The model under review builds one solid part; all positions refer to its coordinate system, in mm. Face numbers are marked on the shaded views. A direction names the side the tool comes from. Give positions to 0.01 mm unless a question says otherwise; leave off trailing zeros. Loops run counter-clockwise (first coordinate to the right, second up) from the corner with the lowest first, then second, coordinate; pieces in that order, holes last. Notation, with made-up numbers: M 26,57 L 53,57 A11 ccw 53,68 Z; hole C 56,-31 d4. An arc over 180 degrees is marked long. Write item = value, one per line. Start each with the question number.
1. We need section A-A on x = 3. Give the boundary of the cut face in (y, z).
2. Wall thickness on line 1 along Y through (x, z) = (2.5, -3.5); line 2 along Z through (x, y) = (6.5, 6.35); line 3 along Y through (x, z) = (10.25, 15.5): over which ranges is each line inside the solid? List them lowest first. Write a range as from..to.
3. Draft analysis for pull direction X (two halves, no side actions). For the marked faces 1, 2 and 3, state which applies: pulls with the +X half, pulls with the -X half, needs draft (parallel to the pull), parting line crosses it, or undercut.
4. For the marked faces 4, 5, 6 and 7, list the 3-axis set-ups (+Z, -Z, +X, -X, +Y, -Y) from which the entire face can be reached by the end or side of a thin tool; tool diameter is ignored.
5. We need section D-D on x = 7. Give the boundary of the cut face in (y, z).
6. We need section C-C on y = 18.5. Give the boundary of the cut face in (x, z).
7. For pin 1 (6.5 mm diameter, centred on x = 6.5, z = -18.14, fed in from -Y); pin 2 (2.5 mm diameter, centred on x = 8, y = 11.5, fed in from +Z); pin 3 (3 mm diameter, centred on x = 3.5, y = -0.5, fed in from -Z), all flat-tipped, find the tip position at first contact; note any pin that passes through.
8. We need section B-B on y = -2. Give the boundary of the cut face in (x, z).
from build123d import *

# Parameters (mm, degrees)
SKETCH2_W           = 29
SKETCH2_H           = 30
SKETCH2_W_2         = 5.4
SKETCH2_H_2         = 3.5
SKETCH2_W_3         = 5.8
SKETCH2_H_3         = 5.3
BOSS_EXTRUDE1_DEPTH = 13
CUT_EXTRUDE1_DEPTH  = 5.3
CUT_EXTRUDE2_DEPTH  = 31
FILLET1_R           = 1


with BuildPart() as part:
    # Sketch2 → Boss-Extrude1 (new body)
    with BuildSketch(Plane(origin=(0, 0, 0), x_dir=(0, 0, -1), z_dir=(1, 0, 0))):
        Rectangle(SKETCH2_W, SKETCH2_H)
        with Locations((-17.2, 5.55)):
            Rectangle(SKETCH2_W_2, SKETCH2_H_2)
        with Locations((4.1, 17.65)):
            Rectangle(SKETCH2_W_3, SKETCH2_H_3)
        with Locations((17.2, 5.55)):
            Rectangle(SKETCH2_W_2, SKETCH2_H_2)
    extrude(amount=BOSS_EXTRUDE1_DEPTH)

    # Sketch3 → Cut-Extrude1 (cut)
    with BuildSketch(Plane(origin=(0, 15, 0), x_dir=(1, 0, 0), z_dir=(0, 1, 0))):
        with BuildLine():
            Line((6.5, 1.2), (9.4, 1.2))
            Line((9.4, 1.2), (9.4, 4.1))
            ThreePointArc((9.4, 4.1), (8.550609665, 2.049390335), (6.5, 1.2))
        make_face()
        with BuildLine():
            ThreePointArc((6.5, 7), (8.550609665, 6.150609665), (9.4, 4.1))
            Line((9.4, 4.1), (9.4, 7))
            Line((9.4, 7), (6.5, 7))
        make_face()
        with BuildLine():
            ThreePointArc((3.6, 4.1), (4.449390335, 6.150609665), (6.5, 7))
            Line((6.5, 7), (3.6, 7))
            Line((3.6, 7), (3.6, 4.1))
        make_face()
        with BuildLine():
            Line((3.6, 1.2), (6.5, 1.2))
            ThreePointArc((6.5, 1.2), (4.449390335, 2.049390335), (3.6, 4.1))
            Line((3.6, 4.1), (3.6, 1.2))
        make_face()
        Polygon((0, 1.2), (3.6, 1.2), (3.6, 4.1), (3.6, 7), (0, 7), align=None)
        Polygon((9.4, 1.2), (13, 1.2), (13, 7), (9.4, 7), (9.4, 4.1), align=None)
        with BuildLine():
            Line((7.75, 19.7), (7.75, 19.9))
            Line((7.75, 19.9), (5.25, 19.9))
            Line((5.25, 19.9), (5.25, 19.7))
            ThreePointArc((5.25, 19.7), (6.5, 16.1387505), (7.75, 19.7))
        make_face()
        with BuildLine():
            Line((5.25, -19.9), (7.75, -19.9))
            Line((7.75, -19.9), (7.75, -19.7))
            ThreePointArc((7.75, -19.7), (6.5, -16.1387505), (5.25, -19.7))
            Line((5.25, -19.7), (5.25, -19.9))
        make_face()
    extrude(amount=CUT_EXTRUDE1_DEPTH, mode=Mode.SUBTRACT)

    # Sketch3<4> → Cut-Extrude2 (cut, through all)
    with BuildSketch(Plane(origin=(0, 15, 0), x_dir=(1, 0, 0), z_dir=(0, 1, 0))):
        with BuildLine():
            Line((7.75, 19.7), (7.75, 19.9))
            Line((7.75, 19.9), (5.25, 19.9))
            Line((5.25, 19.9), (5.25, 19.7))
            ThreePointArc((5.25, 19.7), (6.5, 16.1387505), (7.75, 19.7))
        make_face()
        with BuildLine():
            Line((5.25, -19.9), (7.75, -19.9))
            Line((7.75, -19.9), (7.75, -19.7))
            ThreePointArc((7.75, -19.7), (6.5, -16.1387505), (5.25, -19.7))
            Line((5.25, -19.7), (5.25, -19.9))
        make_face()
    extrude(amount=-CUT_EXTRUDE2_DEPTH, mode=Mode.SUBTRACT)

    # Fillet1
    fillet1_edges = [part.edges().sort_by_distance(p)[0] for p in [
        (0, 5.55, -19.9),
        (0, -5.6, -14.5),
        (0, -15, 0),
        (0, -5.6, 14.5),
        (0, 5.55, 19.9),
        (0, 11.15, 14.5),
        (0, 11.15, -14.5),
        (6.5, -15, -14.5),
        (6.5, -15, 14.5),
        (13, 11.15, 14.5),
        (13, 5.55, 19.9),
        (13, 11.15, -14.5),
        (13, -5.6, 14.5),
        (13, -15, 0),
        (13, -5.6, -14.5),
        (13, 5.55, -19.9),
    ]]
    fillet(fillet1_edges, radius=FILLET1_R)


solid = part.part
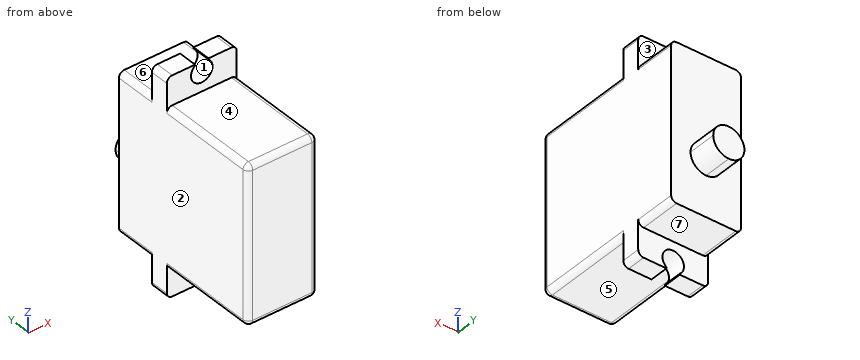
Final values:
q1.outline = M -15,-13.5 A1 ccw -14,-14.5 L 3.8,-14.5 L 3.8,-19.9 L 7.3,-19.9 L 7.3,-14.5 L 15,-14.5 L 15,14.5 L 7.3,14.5 L 7.3,19.9 L 3.8,19.9 L 3.8,14.5 L -14,14.5 A1 ccw -15,13.5 Z
q2.line_1 = -15..15
q2.line_2 = -16.14..16.14
q2.line_3 = 3.8..7.3
q3.face_1 = undercut
q3.face_2 = pulls with the -X half
q3.face_3 = needs draft
q4.face_4 = +Z, +X, -X, -Y
q4.face_5 = -Z, +X, -X, -Y
q4.face_6 = +Z, +X, -X, +Y
q4.face_7 = -Z, +X, -X, +Y
q5.outline = M -15,-13.5 A1 ccw -14,-14.5 L 3.8,-14.5 L 3.8,-16.2 L 7.3,-16.2 L 7.3,-14.5 L 15,-14.5 L 15,-6.96 L 20.3,-6.96 L 20.3,-1.24 L 15,-1.24 L 15,14.5 L 7.3,14.5 L 7.3,16.2 L 3.8,16.2 L 3.8,14.5 L -14,14.5 A1 ccw -15,13.5 Z
q6.outline = C 6.5,-4.1 d5.8
q7.pin_1 = 3.8
q7.pin_2 = 14.5
q7.pin_3 = -14.5
q8.outline = M 0,-13.5 A1 ccw 1,-14.5 L 12,-14.5 A1 ccw 13,-13.5 L 13,13.5 A1 ccw 12,14.5 L 1,14.5 A1 ccw 0,13.5 Z
